```python
from build123d import *

# Parameters (mm, degrees)
F0_W     = 113.6
F0_H     = 38.1
F0_R     = 3.175
F1_DEPTH = 12.7
F2_R     = 15
F3_R     = 9.34
F4_DEPTH = 15.4


with BuildPart() as f1:
    # F0 (on Front) → F1 (new body)
    with BuildSketch(Plane.XZ):
        with Locations((0, 32.391511)):
            Rectangle(F0_W, F0_H)
        with Locations((-50.45, 32.391511)):
            Circle(F0_R, mode=Mode.SUBTRACT)
        with Locations((36.8, 32.391511)):
            Circle(F0_R, mode=Mode.SUBTRACT)
    extrude(amount=F1_DEPTH)

    # F2
    f2_edges = [f1.edges().sort_by_distance(p)[0] for p in [
        (-56.8, -6.35, 51.441511),
        (-56.8, -6.35, 13.341511),
    ]]
    fillet(f2_edges, radius=F2_R)

    # F3 (on face) → F4 (cut)
    with BuildSketch(Plane.XZ.offset(12.7)):
        with Locations((0, 51.177656)):
            Circle(F3_R)
    extrude(amount=-F4_DEPTH, mode=Mode.SUBTRACT)


solid = f1.part
```
Geometry: final body of the model. Coordinates: model frame, mm. Round coordinates to 2 decimals unless told otherwise and drop trailing zeros. Write each loop counter-clockwise with the first axis right and the second up, starting at its lowest first coordinate (ties: lowest second). Pieces come first, ordered by that corner, then holes.
Item 1: Section query B-B (y = -6.5). Return loops of the section in (x, z) (3 decimals), plus the area to 3 significant figures.
Item 2: Section query C-C (x = -50.45). Return loops of the section in (y, z), plus the area to 3 significant figures.
Item 3: Mould query, pull axis X, two halves, no side actions, for faces 1 (the face through (-47.517, -6.261, 31.175)), 2 (the face through (33, -6, 51.442)), 3 (the face through (56.8, -6, 32)). Classes: +X half, -X half, draft (parallel to the pull), parting line (faces both ways), or undercut.
Item 4: Section query D-D (x = 0). Return loops of the section in (y, z).
Item 5: Section query A-A (x = 36.8). Return loops of the section in (y, z).
Item 6: Material intervals for L1, parallel to X at y = -11.25, z = 32; L2, parallel to Z at x = 36.8, y = -4.5; L3, parallel to X at y = -1, z = 48, sorted ascending.
Item 7: Pin query (flat end, axial travel): P1, Ø2, axis at x = 16, z = 33.5, coming from the +Y side. Return the tip coordinate at first contact, or that it passes through.
Completed:
1. outline: (-56.8, 28.342) arc R15 ccw to (-41.8, 13.342) - (56.8, 13.342) - (56.8, 51.442) - (9.336, 51.442) arc R9.34 cw (long way) to (-9.336, 51.442) - (-41.8, 51.442) arc R15 ccw to (-56.8, 36.442) - close; hole circle Ø6.35 at (-50.45, 32.392); hole circle Ø6.35 at (36.8, 32.392)
1. area: 4,030 mm2
2. outline: (-12.7, 16.09) - (0, 16.09) - (0, 29.22) - (-12.7, 29.22) - close; (-12.7, 35.57) - (0, 35.57) - (0, 48.7) - (-12.7, 48.7) - close
2. area: 333 mm2
3. face 1: undercut
3. face 2: draft
3. face 3: +X half
4. outline: (-12.7, 13.34) - (0, 13.34) - (0, 41.84) - (-12.7, 41.84) - close
5. outline: (-12.7, 13.34) - (0, 13.34) - (0, 29.22) - (-12.7, 29.22) - close; (-12.7, 35.57) - (0, 35.57) - (0, 51.44) - (-12.7, 51.44) - close
6. L1: x = -56.8 to -53.6, -47.3 to 33.65, 39.95 to 56.8
6. L2: z = 13.34 to 29.22, 35.57 to 51.44
6. L3: x = -51.36 to -8.78, 8.78 to 56.8
7. P1: stops at y = 0
